Model file for the job. Use its own axes, mm. A direction names the side the tool comes from. Round coordinates to 2 decimals unless told otherwise and drop trailing zeros. Loops run counter-clockwise (first coordinate to the right, second up) from the corner with the lowest first, then second, coordinate; pieces in that order, holes last. Notation, with made-up numbers: M -10.5,-10.75 L 12.5,-10.75 A25 cw 12.5,4.25 Z; hole C 86,-15.75 d8. An arc over 180 degrees is marked long. Answer in a Markdown table with one row per item.
from build123d import *

# Parameters (mm, degrees)
F0_W     = 50
F0_H     = 50
F1_DEPTH = 25
F4_W     = 25
F4_H     = 25
F5_DEPTH = 2.5
F6_R     = 1


with BuildPart() as f1:
    # F0 (on Top) → F1 (new body, symmetric)
    with BuildSketch(Plane.XY):
        Rectangle(F0_W, F0_H)
    extrude(amount=F1_DEPTH, both=True)

    # F4 (on plane+point) → F5 (join)
    with BuildSketch(Plane(origin=(25, 25, -25), x_dir=(-0.8164965809, 0.4082482905, -0.4082482905), z_dir=(0.5773502692, 0.5773502692, -0.5773502692))):
        Rectangle(F4_W, F4_H)
    extrude(amount=-F5_DEPTH)

    # F6
    f6_edges = [f1.edges().sort_by_distance(p)[0] for p in [
        (25, 0, 25),
        (0, 25, 25),
        (-25, 0, 25),
        (0, -25, 25),
        (-25, 25, 0),
        (-25, 0, -25),
        (-25, -25, 0),
        (0, -25, -25),
        (25, -25, 0),
        (-2.165064, 25, -25),
        (25, -2.165064, -25),
        (25, 25, 2.165064),
        (33.762832, 18.453521, -18.453521),
        (23.556624, 14.71779, -32.395459),
        (13.350417, 28.659728, -28.659728),
        (23.556624, 32.395459, -14.71779),
        (34.484519, 28.014043, -10.336374),
        (14.072105, 38.220251, -20.542581),
        (34.484519, 10.336374, -28.014043),
        (14.072105, 20.542581, -38.220251),
    ]]
    fillet(f6_edges, radius=F6_R)


solid = f1.part
1. Pin check, flat tips, straight feed: pin 1 (5 mm diameter, centred on x = 19, y = -7.5, fed in from -Z); pin 2 (8 mm diameter, centred on x = 3, z = 1.5, fed in from +Y); pin 3 (14.5 mm diameter, centred on y = 9, z = -8, fed in from +X). Stop position of each tip, or through.
Verdict:
| item | result |
|---|---|
| pin 1 | stops at z = -25 |
| pin 2 | stops at y = 25 |
| pin 3 | stops at x = 25 |
2. Saw through at A-A (y = -0.5). Write the cut outline in (x, z), and give its area (3 significant figures).
Verdict:
| item | result |
|---|---|
| outline | M -25,-24 A1 ccw -24,-25 L 24,-25 A1 ccw 25,-24 L 25,24 A1 ccw 24,25 L -24,25 A1 ccw -25,24 Z |
| area | 2,500 mm² |
3. Wall check: probe 1 along Z at (x, y) = (24, 8.5). Give the ranges that are in metal, low to high.
Verdict:
| item | result |
|---|---|
| probe 1 | z = -25 to 25 |
4. Tool access for faces 4 (the flat face through (25.775, 22.561, -22.334)), 5 (the cylindrical face through (14.6, 38.178, -20.904)): list every direction of +Z, -Z, +X, -X, +Y, -Y with a clear straight run to the whole face (end or side of a thin tool).
Verdict:
| item | result |
|---|---|
| face 4 | none |
| face 5 | -X, +Y |
5. Mould opens along Y. For faces 1 (the cylindrical face through (34.534, 10.948, -28.2)), 2 (the cylindrical face through (23.6, 32.43, -15.16)), 3 (the cylindrical face through (14.6, 20.904, -38.178)) say: +Y half, -Y half, draft (parallel to the pull), parting line (faces both ways), or undercut.
Verdict:
| item | result |
|---|---|
| face 1 | -Y half |
| face 2 | undercut |
| face 3 | parting line |
